Job drawing, mm, ordinate dimensions from the low corner. One solid piece. Give positions to 0.01 mm unless a question says otherwise; leave off trailing zeros. Order: outer loops, then holes, each group sorted by start corner. A loop starts at its lowest first (then second) coordinate and runs counter-clockwise, first axis right, second up. Notation, with made-up numbers: M 45.25,76.5 L 79.25,76.5 A11 ccw 79.25,89.5 Z; hole C -7,8 d10. An arc over 180 degrees is marked long. One line per item, written item: value. Start each with the question number.
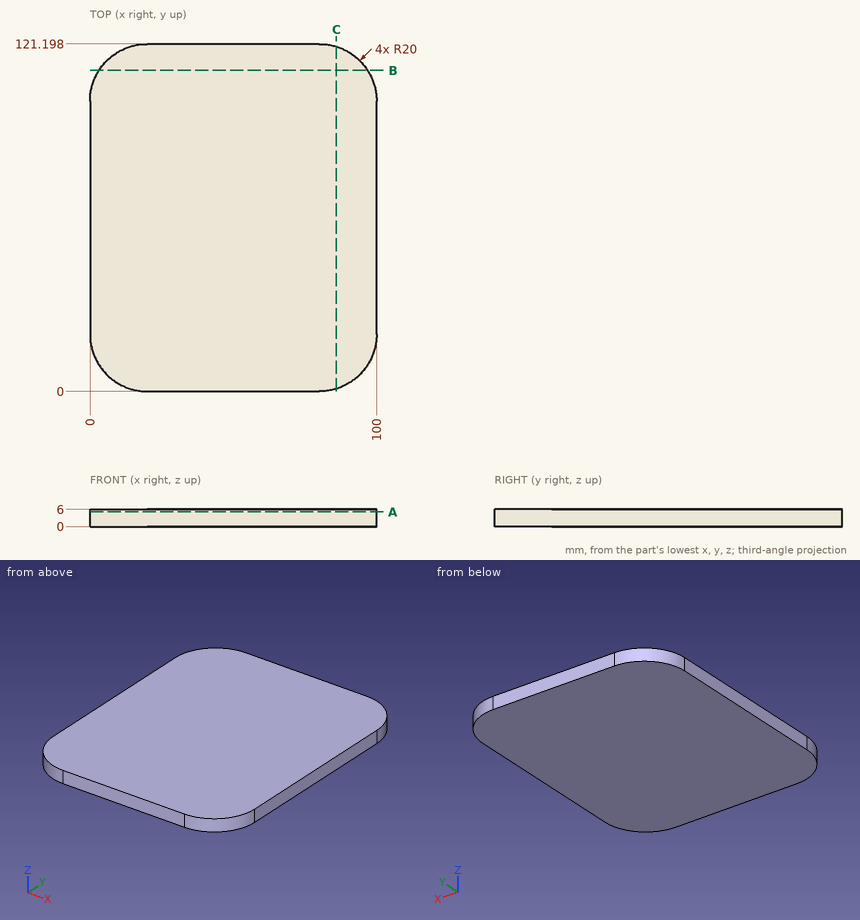
1) Drop a flat-ended pin along its axis: P1, Ø3, axis at x = 39.5, y = 21, coming from the -Z side. Give the stop position or say it passes through.
2) Slice it at B-B (y = 112). List the corners of the cut face in (x, z), plus the area to 3 significant figures.
3) Slice it at C-C (x = 86). List the corners of the cut face in (y, z).
4) Drill centre lines: line 1 (Y direction, x = 84, z = 5.25) (1 decimal); line 2 (Y direction, x = 82.5, z = 1.6). Where is each one in solid material? Low to high.
5) Slice it at A-A (z = 5.1). List the corners of the cut face in (x, y), plus the area to 3 significant figures.
Results list:
1. P1: stops at z = 0
2. outline: M 3.17,0 L 96.83,0 L 96.83,6 L 3.17,6 Z
2. area: 562 mm²
3. outline: M 0.92,0 L 120.28,0 L 120.28,6 L 0.92,6 Z
4. line 1: y = 0.4 to 120.8
4. line 2: y = 0.16 to 121.04
5. outline: M 0,20 A20 ccw 20,0 L 80,0 A20 ccw 100,20 L 100,101.2 A20 ccw 80,121.2 L 20,121.2 A20 ccw 0,101.2 Z
5. area: 11,800 mm²
